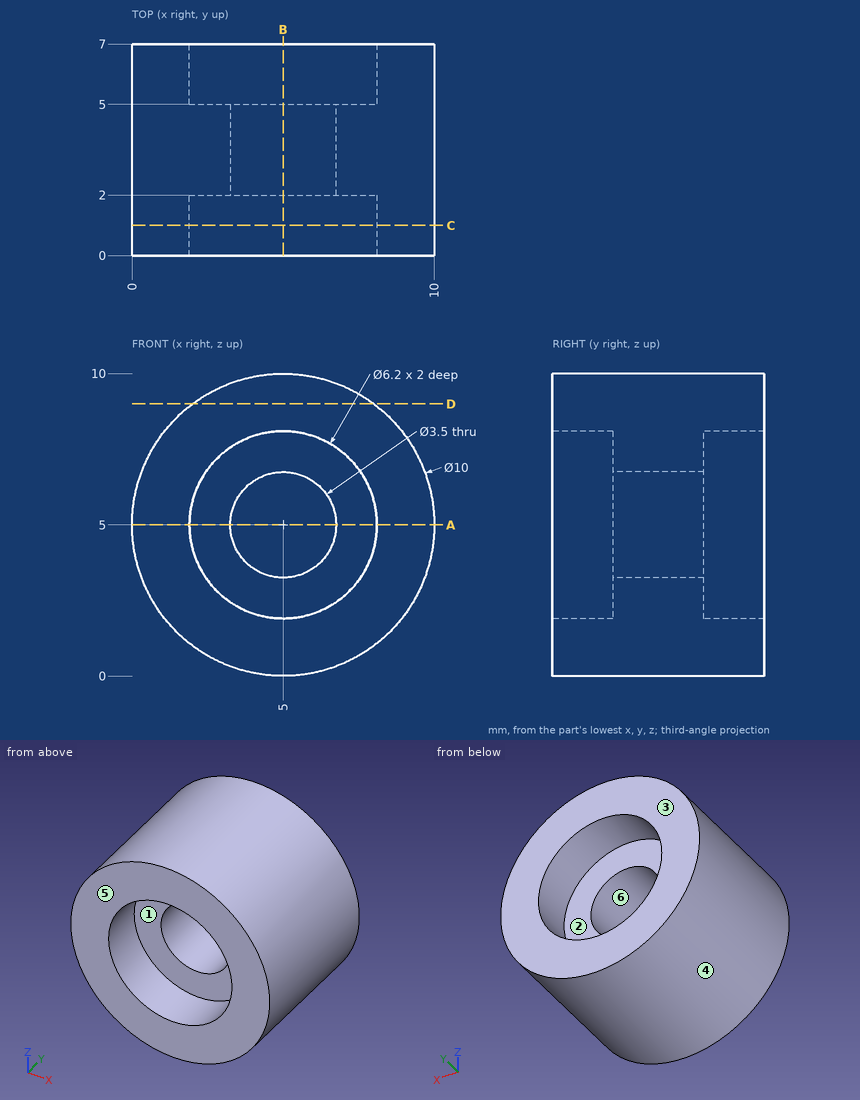
Can you work these out from the drawing? Everything is in mm from the part's minimum corner. A direction names the side the tool comes from. Coordinates: 2 decimals unless noted, no trailing zeros. Loops run counter-clockwise (first coordinate to the right, second up) from the corner with the lowest first, then second, coordinate; pieces in that order, holes last.
1. If we mould it in two halves opening along X, with no side actions, what happens to the marked faces 4, 5 and 6? For each: pulls with the +X half, pulls with the -X half, needs draft (parallel to the pull), parting line crosses it, or undercut.
2. Imagine slicing it at A-A, the plane z = 5. Please give me the cut outline in (x, y).
3. For the marked faces 1, 2 and 3, which set-ups out of +Z, -Z, +X, -X, +Y, -Y let a thin tool reach every point of the face, with its end or its side?
4. Imagine slicing it at D-D, the plane z = 9. Please give me the cut outline in (x, y), and give its area (3 significant figures).
5. I need wall thicknesses on L1, parallel to Z at x = 5, y = 2.95; L2, parallel to Z at x = 5, y = 0.5; L3, parallel to X at y = 2.75, z = 4.25. Which ranges of each line are inside material? Lowest first, please.
6. Imagine slicing it at C-C, the plane y = 1. Please give me the cut outline in (x, z), and give its area (3 significant figures).
7. Imagine slicing it at B-B, the plane x = 5. Please give me the cut outline in (y, z).
8. For P1, Ø2, axis at x = 1, y = 2, coming from the +Z side; P2, Ø1, axis at x = 9, y = 3, coming from the +Z side; P3, Ø5.5, axis at x = 5, z = 5, coming from the +Y side; P4, Ø2, axis at x = 5, z = 5, coming from the +Y side, each with a flat end and sliding along its axis, tell me the tip position at first contact or that it passes through.
Taken from the geometry:
1. face 4: parting line crosses it
1. face 5: needs draft
1. face 6: undercut
2. outline: (0, 0) - (1.9, 0) - (1.9, 2) - (3.25, 2) - (3.25, 5) - (1.9, 5) - (1.9, 7) - (0, 7) - close; (6.75, 2) - (8.1, 2) - (8.1, 0) - (10, 0) - (10, 7) - (8.1, 7) - (8.1, 5) - (6.75, 5) - close
3. face 1: -Y
3. face 2: +Y
3. face 3: +Z, -Z, +X, -X, +Y
4. outline: (2, 0) - (8, 0) - (8, 7) - (2, 7) - close
4. area: 42.0 mm2
5. L1: z = 0 to 3.25, 6.75 to 10
5. L2: z = 0 to 1.9, 8.1 to 10
5. L3: x = 0.06 to 3.42, 6.58 to 9.94
6. outline: circle Ø10 at (5, 5); hole circle Ø6.2 at (5, 5)
6. area: 48.3 mm2
7. outline: (0, 0) - (7, 0) - (7, 1.9) - (5, 1.9) - (5, 3.25) - (2, 3.25) - (2, 1.9) - (0, 1.9) - close; (0, 8.1) - (2, 8.1) - (2, 6.75) - (5, 6.75) - (5, 8.1) - (7, 8.1) - (7, 10) - (0, 10) - close
8. P1: stops at z = 9
8. P2: stops at z = 8.57
8. P3: stops at y = 5
8. P4: passes through
